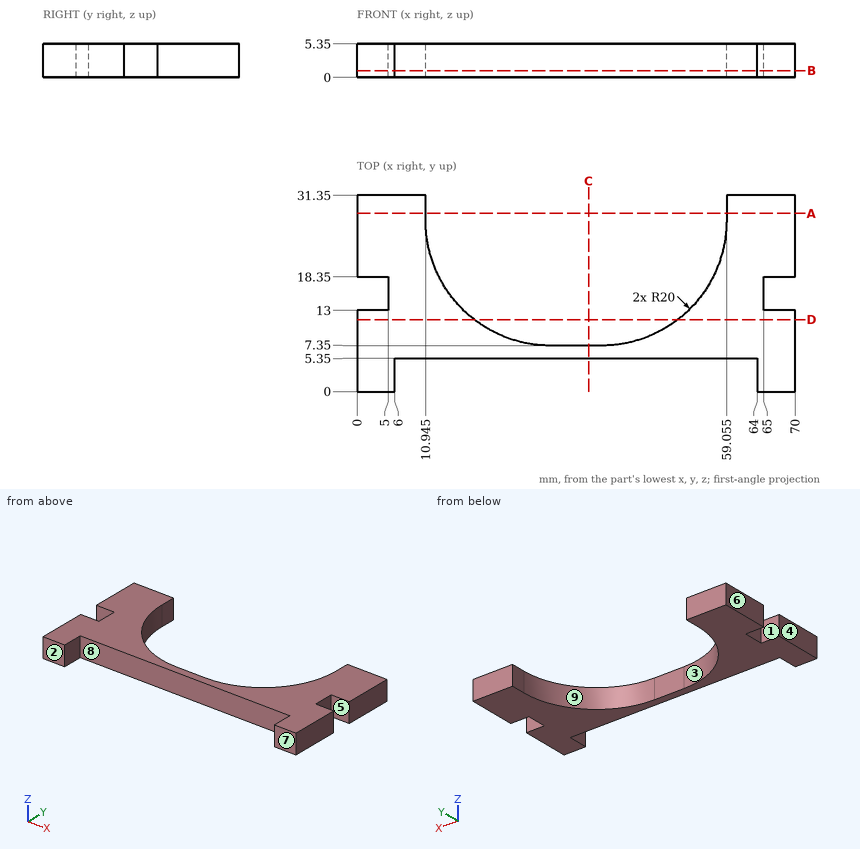
Geometry check sheet. Reference: drawing and pictorial views, mm from the part's lowest x, y, z. A direction names the side the tool comes from. Coordinates: 2 decimals unless noted, no trailing zeros. Order: outer loops, then holes, each group sorted by start corner. A loop starts at its lowest first (then second) coordinate and runs counter-clockwise, first axis right, second up.
Item 1: Section check A-A, the plane y = 28.5. Enter the section's corners in (x, z) (3 decimals).
Filled in:
outline: (0, 0) - (10.945, 0) - (10.945, 5.35) - (0, 5.35) - close; (59.055, 0) - (70, 0) - (70, 5.35) - (59.055, 5.35) - close
Item 2: Depth check by flat-ended pin: pin 1 (1.6 mm diameter, centred on y = 15.5, z = 3.5, fed in from +X); pin 2 (2.5 mm diameter, centred on x = 36.5, z = 3.5, fed in from +Y). Enter the tip coordinate at first touch or a pass-through.
Filled in:
pin 1: stops at x = 65
pin 2: stops at y = 7.35
Item 3: Section check D-D, the plane y = 11.5. Enter the section's corners in (x, z).
Filled in:
outline: (0, 0) - (18.75, 0) - (18.75, 5.35) - (0, 5.35) - close; (51.25, 0) - (70, 0) - (70, 5.35) - (51.25, 5.35) - close
Item 4: Material ranges on L1, parallel to Y at x = 4.5, z = 4.2; L2, parallel to X at y = 29.5, z = 0.7 (3 decimals); L3, parallel to X at y = 3, z = 3.1, recorded low to high.
Filled in:
L1: y = 0 to 13, 18.35 to 31.35
L2: x = 0 to 10.945, 59.055 to 70
L3: x = 0 to 6, 64 to 70
Item 5: Access from +Z, -Z, +X, -X, +Y, -Y to the whole of each face (thin tool, end or side, straight path). Record for the marked faces 1, 2, 3, 4 and 5.
Filled in:
face 1: +Z, -Z, -X
face 2: +Z, -Z, +X, -X, -Y
face 3: +Z, -Z, +Y
face 4: +Z, -Z, -X, +Y, -Y
face 5: +Z, -Z, +X
Item 6: Section check B-B, the plane z = 1.1. Enter the section's corners in (x, y) (3 decimals), then the cut area to 3 significant figures.
Filled in:
outline: (0, 0) - (6, 0) - (6, 5.35) - (64, 5.35) - (64, 0) - (70, 0) - (70, 13) - (65, 13) - (65, 18.35) - (70, 18.35) - (70, 31.35) - (59.055, 31.35) - (59.055, 27.35) arc R20 cw to (39.055, 7.35) - (30.945, 7.35) arc R20 cw to (10.945, 27.35) - (10.945, 31.35) - (0, 31.35) - (0, 18.35) - (5, 18.35) - (5, 13) - (0, 13) - close
area: 848 mm2
Item 7: Section check C-C, the plane x = 37. Enter the section's corners in (y, z).
Filled in:
outline: (5.35, 0) - (7.35, 0) - (7.35, 5.35) - (5.35, 5.35) - close
Item 8: Release check for a two-part mould opening along X. For the marked faces 6, 7, 8 and 9 record: +X half, -X half, draft (parallel to the pull), parting line (faces both ways), or undercut.
Filled in:
face 6: -X half
face 7: draft
face 8: undercut
face 9: undercut
